Could you check a few things on this drawing? It's one solid part, dimensions in mm from its lowest x, y, z. Give positions to 0.01 mm unless a question says otherwise; leave off trailing zeros. Order: outer loops, then holes, each group sorted by start corner. A loop starts at its lowest first (then second) coordinate and runs counter-clockwise, first axis right, second up.
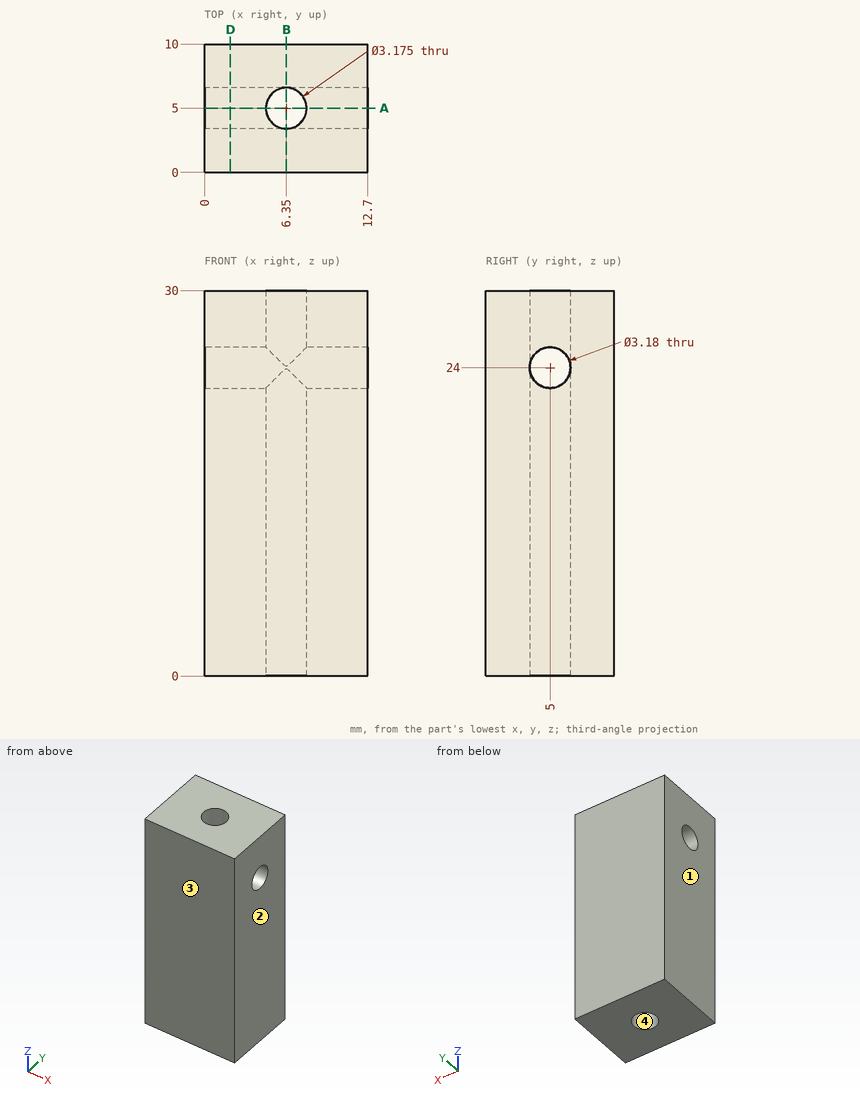
Item 1: For pin 1 (5 mm diameter, centred on x = 7.5, y = 4, fed in from -Z), with a flat end and sliding along its axis, tell me the tip position at first contact or that it passes through.
Findings:
pin 1: stops at z = 0
Item 2: Please list where these lines run through material, in increasing order: line 1 along X through (y, z) = (5, 26.85); line 2 along Y through (x, z) = (6.35, 14.5); line 3 along Y through (x, z) = (7.75, 6.5).
Findings:
line 1: x = 0 to 4.76, 7.94 to 12.7
line 2: y = 0 to 3.41, 6.59 to 10
line 3: y = 0 to 4.25, 5.75 to 10
Item 3: Imagine slicing it at B-B on x = 6.35. List the corners of the cut face in (y, z) for me.
Findings:
outline: (0, 0) - (3.41, 0) - (3.41, 23.91) arc R1.59 cw to (3.41, 24.09) - (3.41, 30) - (0, 30) - close; (6.59, 0) - (10, 0) - (10, 30) - (6.59, 30) - (6.59, 24.09) arc R1.59 cw to (6.59, 23.91) - close
Item 4: Imagine slicing it at D-D on x = 2. List the corners of the cut face in (y, z) for me.
Findings:
outline: (0, 0) - (10, 0) - (10, 30) - (0, 30) - close; hole circle Ø3.18 at (5, 24)
Item 5: Imagine slicing it at A-A on y = 5. List the corners of the cut face in (x, z) for me, then the cut area to 3 significant figures.
Findings:
outline: (0, 0) - (4.76, 0) - (4.76, 22.41) - (0, 22.41) - close; (0, 25.59) - (4.76, 25.59) - (4.76, 30) - (0, 30) - close; (7.94, 0) - (12.7, 0) - (12.7, 22.41) - (7.94, 22.41) - close; (7.94, 25.59) - (12.7, 25.59) - (12.7, 30) - (7.94, 30) - close
area: 255 mm2
Item 6: We'd pull the mould along X, two halves only. Please class the marked faces 1, 2, 3 and 4: +X half, -X half, draft (parallel to the pull), parting line (faces both ways), or undercut.
Findings:
face 1: -X half
face 2: +X half
face 3: draft
face 4: undercut
